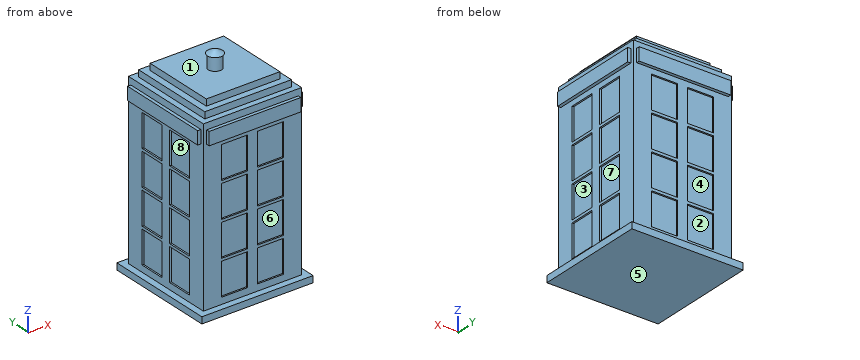
```python
from build123d import *

# Parameters (mm, degrees)
F0_W             = 107.95
F0_H             = 107.95
F1_DEPTH         = 6.35
F2_W             = 95.25
F2_H             = 95.25
F3_DEPTH         = 165.1
F4_W             = 84.073998034
F4_H             = 84.073998034
F5_DEPTH         = 6.35
F6_W             = 71.373998034
F6_H             = 71.373998034
F7_DEPTH         = 6.35
F8_W             = 88.9
F8_H             = 12.7
F9_DEPTH         = 3.175
F9_COPIES_COUNT  = 4
F11_R            = 6.35
F12_DEPTH        = 12.7
F13_R            = 7.366000209
F14_DEPTH        = 25.4
F14_TAPER        = 60
F15_W            = 25.4
F15_H            = 31.75
F16_DEPTH        = 1.5875
F16_COPIES_COUNT = 4


# Not quite as in the source:
# - a pattern or mirror of a feature is missing from the dataset's text; its kind, count and spacing are read off the source's solid


with BuildPart() as f1:
    # F0 (on Top) → F1 (new body)
    with BuildSketch(Plane.XY):
        Rectangle(F0_W, F0_H)
    extrude(amount=F1_DEPTH)

    # F2 (on face) → F3 (join)
    with BuildSketch(Plane.XY.offset(6.35)):
        Rectangle(F2_W, F2_H)
    extrude(amount=F3_DEPTH)

    # F4 (on face) → F5 (join)
    with BuildSketch(Plane.XY.offset(171.45)):
        Rectangle(F4_W, F4_H)
    extrude(amount=F5_DEPTH)

    # F6 (on face) → F7 (join)
    with BuildSketch(Plane.XY.offset(177.8)):
        Rectangle(F6_W, F6_H)
    extrude(amount=F7_DEPTH)

    # F8 (on face) → F9 (join)
    with BuildSketch(Plane(origin=(-47.625, 0, 0), x_dir=(0, -1, 0), z_dir=(-1, 0, 0))):
        with Locations((0, 158.7718427181)):
            Rectangle(F8_W, F8_H)
    f9 = extrude(amount=F9_DEPTH)

    # F9_copies: F9 ×4 about axis
    f9_copies_axis = Axis((0, 0, 0), (0, 0, 1))
    for i in range(1, F9_COPIES_COUNT):
        add(f9.rotate(f9_copies_axis, i * 360 / F9_COPIES_COUNT))

    # F11 (on face) → F12 (join)
    with BuildSketch(Plane.XY.offset(184.15)):
        Circle(F11_R)
    extrude(amount=F12_DEPTH)

    # F13 (on face) → F14 (join)
    with BuildSketch(Plane.XY.offset(196.85)):
        Circle(F13_R)
    extrude(amount=F14_DEPTH, taper=F14_TAPER)

    # F15 (on face) → F16 (cut)
    with BuildSketch(Plane.XZ.offset(47.625)):
        with Locations((-17.4625, 28.575)):
            Rectangle(F15_W, F15_H)
        with Locations((-17.4625, 62.865)):
            Rectangle(F15_W, F15_H)
        with Locations((-17.4625, 97.155)):
            Rectangle(F15_W, F15_H)
        with Locations((-17.4625, 131.445)):
            Rectangle(F15_W, F15_H)
        with Locations((17.4625, 97.155)):
            Rectangle(F15_W, F15_H)
        with Locations((17.4625, 131.445)):
            Rectangle(F15_W, F15_H)
        with Locations((17.4625, 62.865)):
            Rectangle(F15_W, F15_H)
        with Locations((17.4625, 28.575)):
            Rectangle(F15_W, F15_H)
    f16 = extrude(amount=-F16_DEPTH, mode=Mode.SUBTRACT)

    # F16_copies: F16 ×4 about axis
    f16_copies_axis = Axis((0, 0, 0), (0, 0, 1))
    for i in range(1, F16_COPIES_COUNT):
        add(f16.rotate(f16_copies_axis, i * 360 / F16_COPIES_COUNT), mode=Mode.SUBTRACT)


solid = f1.part
```
Source: CAD feature listing. Evaluate the final solid. Frame: model axes, mm. Face numbers are marked on the shaded views. A direction names the side the tool comes from. Give positions to 0.01 mm unless a question says otherwise; leave off trailing zeros. Put each result on its own line as item: value. Start each with the question number.
1) Reachability of the marked faces 4, 5, 6, 7 and 8 from +Z, -Z, +X, -X, +Y, -Y: full face, straight path, thin tool, end or side. Return the list, or none.
2) Material intervals for probe 1 along Z at (x, y) = (-34, -48.5); probe 2 along X at (y, z) = (31, 70.5) (3 decimals); probe 3 along Z at (x, y) = (-44, 3), sorted ascending.
3) Draft query along Y for the marked faces 1, 2 and 3. Return one class per face: released by +Y, released by -Y, zero draft, split by the parting line, or undercut.
4) Contact query for flat-ended pins moving along their axis: P1, Ø3, axis at y = -1.5, z = 165, coming from the +X side; P2, Ø1.5, axis at y = -23.5, z = 179, coming from the +X side; P3, Ø1.7, axis at x = -22, y = 47, coming from the +Z side. Output: stop coordinate, or through.
Results are:
1. face 4: +Y
1. face 5: -Z, +X, -X, +Y, -Y
1. face 6: -Y
1. face 7: +X
1. face 8: -X
2. probe 1: z = 0 to 6.35, 152.42 to 165.12
2. probe 2: x = -47.625 to 47.625
2. probe 3: z = 0 to 171.45
3. face 1: zero draft
3. face 2: released by +Y
3. face 3: undercut
4. P1: stops at x = 50.8
4. P2: stops at x = 35.69
4. P3: stops at z = 171.45
